Input: part model. Units: mm. Frame: model coordinates. Face numbers are marked on the shaded views. A direction names the side the tool comes from. Give positions to 0.01 mm unless a question says otherwise; leave off trailing zeros. Loops run counter-clockwise (first coordinate to the right, second up) from the corner with the lowest first, then second, coordinate; pieces in that order, holes last. Notation, with made-up numbers: (15.5, 82.5) - (59.5, 82.5) arc R5 cw to (59.5, 89.5) - close; hole circle Ø1 at (29, -31.5). An arc over 180 degrees is marked (long way). One line per question, with ' | ' between items. Start each with the question number.
from build123d import *

# Parameters (mm, degrees)
SKETCH_W        = 52
SKETCH_H        = 68
PAD_DEPTH       = 17
SKETCH001_W     = 48.5
SKETCH001_H     = 64.5
POCKET_DEPTH    = 16
SKETCH002_R     = 1.75
PAD001_DEPTH    = 4.55
SKETCH003_R     = 1.3
PAD002_DEPTH    = 6.55
SKETCH004_W     = 4
SKETCH004_H     = 2
POCKET001_DEPTH = 5
POCKET002_DEPTH = 5
SKETCH006_R     = 2.75
SKETCH006_W     = 12
SKETCH006_H     = 1.5
SKETCH006_W_2   = 15
POCKET003_DEPTH = 5
SKETCH007_R     = 1
SKETCH007_W     = 14.5
SKETCH007_H     = 1.5
POCKET004_DEPTH = 5
POCKET006_DEPTH = 1
SKETCH008_W     = 5.1
SKETCH008_H     = 1.3
POCKET007_DEPTH = 1.3
CHAMFER_SIZE    = 1
FILLET_R        = 1.5


with BuildPart() as part:
    # Sketch → Pad (new body)
    with BuildSketch(Plane.XY):
        with Locations((24.25, 32.25)):
            Rectangle(SKETCH_W, SKETCH_H)
    extrude(amount=PAD_DEPTH)

    # Sketch001 → Pocket (cut)
    with BuildSketch(Plane.XY.offset(17)):
        with Locations((24.25, 32.25)):
            Rectangle(SKETCH001_W, SKETCH001_H)
    extrude(amount=-POCKET_DEPTH, mode=Mode.SUBTRACT)

    # Sketch002 (on Face11 of Pocket) → Pad001 (join)
    with BuildSketch(Plane.XY.offset(1)):
        with Locations((3.05, 3.05)):
            Circle(SKETCH002_R)
        with Locations((3.05, 61.05)):
            Circle(SKETCH002_R)
        with Locations((45.05, 3.05)):
            Circle(SKETCH002_R)
        with Locations((45.05, 61.05)):
            Circle(SKETCH002_R)
    extrude(amount=PAD001_DEPTH)

    # Sketch003 (on Face11 of Pad001) → Pad002 (join)
    with BuildSketch(Plane.XY.offset(1)):
        with Locations((3.05, 61.05)):
            Circle(SKETCH003_R)
        with Locations((45.05, 61.05)):
            Circle(SKETCH003_R)
        with Locations((3.05, 3.05)):
            Circle(SKETCH003_R)
        with Locations((45.05, 3.05)):
            Circle(SKETCH003_R)
    extrude(amount=PAD002_DEPTH)

    # Sketch004 (on Face2 of Pad002) → Pocket001 (cut)
    with BuildSketch(Plane(origin=(-1.75, 0, 0), x_dir=(0, -1, 0), z_dir=(-1, 0, 0))):
        with BuildLine():
            ThreePointArc((-28.6, 11.1), (-30.7, 9), (-28.6, 6.9))
            Line((-28.6, 6.9), (-23.4, 6.9))
            ThreePointArc((-23.4, 6.9), (-21.3, 9), (-23.4, 11.1))
            Line((-28.6, 11.1), (-23.4, 11.1))
        make_face()
        with BuildLine():
            ThreePointArc((-13.6, 11.1), (-15.7, 9), (-13.6, 6.9))
            Line((-13.6, 6.9), (-8.4, 6.9))
            ThreePointArc((-8.4, 6.9), (-6.3, 9), (-8.4, 11.1))
            Line((-13.6, 11.1), (-8.4, 11.1))
        make_face()
        with Locations((-44.5, 7)):
            Rectangle(SKETCH004_W, SKETCH004_H)
    extrude(amount=-POCKET001_DEPTH, mode=Mode.SUBTRACT)

    # Sketch005 (on Face2 of Pocket001) → Pocket002 (cut)
    with BuildSketch(Plane(origin=(-1.75, 0, 0), x_dir=(0, -1, 0), z_dir=(-1, 0, 0))):
        Polygon((-56, 10.6), (-49, 10.6), (-49, 7.85), (-49.75, 7.1), (-55.25, 7.1), (-56, 7.85), align=None)
    extrude(amount=-POCKET002_DEPTH, mode=Mode.SUBTRACT)

    # Sketch006 (on Face1 of Pocket002) → Pocket003 (cut)
    with BuildSketch(Plane(origin=(0, 66.25, 0), x_dir=(-1, 0, 0), z_dir=(0, 1, 0))):
        with Locations((-13.3, 9.85)):
            Circle(SKETCH006_R)
        with Locations((-22.7, 3.75)):
            Rectangle(SKETCH006_W, SKETCH006_H)
        with Locations((-33.5, 7.85)):
            Rectangle(SKETCH006_W_2, SKETCH006_H)
    extrude(amount=-POCKET003_DEPTH, mode=Mode.SUBTRACT)

    # Sketch007 (on Face15 of Pocket007) → Pocket004 (cut)
    with BuildSketch(Plane.XZ.offset(1.75)):
        with Locations((7.75, 8.1)):
            Circle(SKETCH007_R)
        with Locations((24.25, 7.85)):
            Rectangle(SKETCH007_W, SKETCH007_H)
        with BuildLine():
            ThreePointArc((36.5, 11.1), (35.5, 10.1), (36.5, 9.1))
            Line((36.5, 9.1), (41, 9.1))
            ThreePointArc((41, 9.1), (42, 10.1), (41, 11.1))
            Line((36.5, 11.1), (41, 11.1))
        make_face()
    extrude(amount=-POCKET004_DEPTH, mode=Mode.SUBTRACT)

    # Sketch009 → Pocket006 (cut)
    with BuildSketch(Plane.YZ.offset(50.25)):
        with BuildLine():
            Line((22.3, 16), (42.2, 16))
            ThreePointArc((42.2, 15), (42.7, 15.5), (42.2, 16))
            Line((42.2, 15), (22.3, 15))
            ThreePointArc((22.3, 16), (21.8, 15.5), (22.3, 15))
        make_face()
    extrude(amount=-POCKET006_DEPTH, mode=Mode.SUBTRACT)

    # Sketch008 (on Face34 of Pocket006) → Pocket007 (cut)
    with BuildSketch(Plane.YZ):
        with Locations((24.7, 15.1)):
            Rectangle(SKETCH008_W, SKETCH008_H)
        with Locations((39.8, 15.1)):
            Rectangle(SKETCH008_W, SKETCH008_H)
    extrude(amount=-POCKET007_DEPTH, mode=Mode.SUBTRACT)

    # Chamfer
    chamfer_edges = [part.edges().sort_by_distance(p)[0] for p in [
        (-1.75, 49.375, 7.475),
        (-1.75, 49, 9.225),
        (-1.75, 52.5, 10.6),
        (-1.75, 56, 9.225),
        (-1.75, 55.625, 7.475),
        (-1.75, 52.5, 7.1),
        (-1.75, 46.5, 7),
        (-1.75, 44.5, 8),
        (-1.75, 42.5, 7),
        (-1.75, 44.5, 6),
        (16.05, 66.25, 9.85),
    ]]
    chamfer(chamfer_edges, length=CHAMFER_SIZE)

    # Fillet
    fillet_edges = [part.edges().sort_by_distance(p)[0] for p in [
        (-1.75, 66.25, 8.5),
        (-1.75, 32.25, 0),
        (24.25, 66.25, 0),
        (-1.75, -1.75, 8.5),
        (24.25, -1.75, 0),
        (50.25, -1.75, 8.5),
        (50.25, 32.25, 0),
        (50.25, 66.25, 8.5),
    ]]
    fillet(fillet_edges, radius=FILLET_R)


solid = part.part
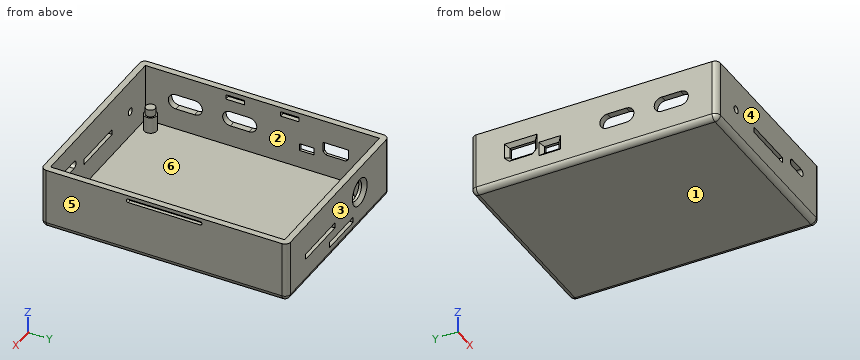
Q1. Section B-B, the plane x = 39. Output: boundary loops of the cut face in (y, z), plus the area to 3 significant figures.
Q2. Section C-C, the plane x = 7.75. Output: boundary loops of the cut face in (y, z), plus the area to 3 significant figures.
Q3. Access query for the marked faces 5 and 6. Directions: +Z, -Z, +X, -X, +Y, -Y. A direction counts if a zero-diameter tool reaches every point of the face in a straight line with its end or side. Return the directions, or none.
Q4. Section D-D, the plane x = 32.5. Output: boundary loops of the cut face in (y, z).
Q5. Line query: L1, parallel to Y at x = 42, z = 9.75; L2, parallel to X at y = 7, z = 5.5; L3, parallel to X at y = 44, z = 6.75. Output: solid intervals per line, ascending. Write a range as from..to.
Q6. Section A-A, the plane y = 26. Output: boundary loops of the cut face in (x, z).
Q7. Draft query along Y for the marked faces 1, 2, 3 and 4. Return one class per face: +Y half, -Y half, draft (parallel to the pull), parting line (faces both ways), or undercut.
Q8. First-contact query: pin 1 (0.8 mm diameter, centred on x = 3, y = 60.5, fed in from +Z); pin 2 (1.6 mm diameter, centred on y = -1, z = 7.5, fed in from +X); pin 3 (12 mm diameter, centred on x = 17, y = 53, fed in from +Z); pin 4 (1.1 mm diameter, centred on x = 50, y = 28.5, fed in from -Z). Flat tips, straight axial feed; report the tip coordinate or a pass-through.
Solved:
1) outline: (-1.75, 1.5) arc R1.5 ccw to (-0.25, 0) - (64.75, 0) arc R1.5 ccw to (66.25, 1.5) - (66.25, 7.1) - (64.5, 7.1) - (64.5, 1) - (0, 1) - (0, 9.1) - (-1.75, 9.1) - close; (-1.75, 11.1) - (0, 11.1) - (0, 17) - (-1.75, 17) - close; (64.5, 8.6) - (66.25, 8.6) - (66.25, 17) - (64.5, 17) - close | area: 117 mm²
2) outline: (-1.75, 1.5) arc R1.5 ccw to (-0.25, 0) - (64.75, 0) arc R1.5 ccw to (66.25, 1.5) - (66.25, 17) - (64.5, 17) - (64.5, 1) - (0, 1) - (0, 7.1) - (-1.75, 7.1) - close; (-1.75, 9.1) - (0, 9.1) - (0, 17) - (-1.75, 17) - close | area: 120 mm²
3) face 5: +Z, -Z, +X, +Y, -Y | face 6: +Z
4) outline: (-1.75, 1.5) arc R1.5 ccw to (-0.25, 0) - (64.75, 0) arc R1.5 ccw to (66.25, 1.5) - (66.25, 7.1) - (64.5, 7.1) - (64.5, 1) - (0, 1) - (0, 17) - (-1.75, 17) - close; (64.5, 8.6) - (66.25, 8.6) - (66.25, 17) - (64.5, 17) - close
5) L1: y = -1.75..0, 64.5..66.25 | L2: x = -1.75..0, 48.5..50.25 | L3: x = 48.5..50.25
6) outline: (-1.75, 1.5) arc R1.5 ccw to (-0.25, 0) - (48.75, 0) arc R1.5 ccw to (50.25, 1.5) - (50.25, 15) - (49.25, 15) - (49.25, 16) - (50.25, 16) - (50.25, 17) - (48.5, 17) - (48.5, 1) - (0, 1) - (0, 6.9) - (-1.75, 6.9) - close; (-1.75, 11.1) - (0, 11.1) - (0, 14.45) - (-1.3, 14.45) - (-1.3, 15.75) - (0, 15.75) - (0, 17) - (-1.75, 17) - close
7) face 1: draft | face 2: undercut | face 3: +Y half | face 4: -Y half
8) pin 1: stops at z = 7.55 | pin 2: stops at x = 50.25 | pin 3: stops at z = 1 | pin 4: stops at z = 0.17
